Part model, mm, in its own coordinate system. Face numbers are marked on the shaded views. A direction names the side the tool comes from. Give positions to 0.01 mm unless a question says otherwise; leave off trailing zeros. Write each loop counter-clockwise with the first axis right and the second up, starting at its lowest first coordinate (ties: lowest second). Pieces come first, ordered by that corner, then holes. Notation, with made-up numbers: M 70,2 L 89,2 A14 ccw 89,26 Z; hole C -15.75,42 d5. An arc over 180 degrees is marked long. Answer as CSV lines item,"result". Start each with the question number.
Item 1: Band-saw the part on B-B, the plane z = 23. List the corners of the cut face in (x, y), then the cut area to 3 significant figures.
Item 2: Band-saw the part on D-D, the plane z = 9. List the corners of the cut face in (x, y), then the cut area to 3 significant figures.
Item 3: Band-saw the part on C-C, the plane x = 22.5. List the corners of the cut face in (y, z).
Item 4: Wall check: L1, parallel to Y at x = 39, z = 1; L2, parallel to Y at x = 28, z = 8; L3, parallel to Y at x = 44.5, z = 46.5. Give the ranges that are in metal, low to high. Write a range as from..to.
Item 5: Two-plate mould, pull along Y, no slides. Class the marked faces 5, 6 and 7: +Y half, -Y half, draft (parallel to the pull), parting line (faces both ways), or undercut.
Item 6: Pin check, flat tips, straight feed: pin 1 (16 mm diameter, centred on x = 12, z = 23, fed in from -Y); pin 2 (4.5 mm diameter, centred on x = 19.5, y = 24.5, fed in from +Z); pin 3 (1 mm diameter, centred on x = 43.5, y = 31, fed in from +Z). Stop position of each tip, or through.
Item 7: 3-axis set-ups, long thin cutter, end or side, ignore diameter. For the marked faces 1, 2, 3 and 4: which of +Z, -Z, +X, -X, +Y, -Y reach the whole face in a straight line?
Item 8: Band-saw the part on A-A, the plane y = 58. List the corners of the cut face in (x, z).
from build123d import *

# Parameters (mm, degrees)
F0_W           = 56
F0_H           = 66
F1_DEPTH       = 4
F3_D           = 7
F4_SIZE2       = 10
F4_SIZE        = 10
F5_SIZE2       = 16
F5_SIZE        = 16
F8_DEPTH       = 10
F8_DEPTH_BACK  = 10
F9_R           = 2
F11_R          = 5
F11_R_2        = 4
F12_DEPTH      = 20
F11_R_3        = 9.5
F13_DEPTH      = 1
F13_DEPTH_BACK = 21
F15_DEPTH      = 8
F15_DEPTH_BACK = 28
F10_W          = 12
F10_H          = 50
F16_DEPTH      = 61.001
F18_T4_DEPTH   = 56
F18_T9_DEPTH   = 61
F18_T15_DEPTH  = 56
F18_T20_DEPTH  = 61
F18_T26_DEPTH  = 56
F18_T31_DEPTH  = 61
F18_T37_DEPTH  = 56
F18_T42_DEPTH  = 61
F19_R          = 2


# Not quite as in the source:
# - a fillet or chamfer that OpenCascade refuses, or shapes differently, is made with other operations: its cross-section is extruded or revolved along the edge and cut away or added


with BuildPart() as f1:
    # F0 (on Top) → F1 (new body)
    with BuildSketch(Plane.XY):
        with Locations((28, 33)):
            Rectangle(F0_W, F0_H)
    extrude(amount=F1_DEPTH)

    # F3 (through all)
    with Locations(Plane.XY.offset(4)):
        with Locations((12, 58), (39, 58), (39, 8), (12, 8)):
            Hole(F3_D / 2)

    # F4
    f4_edges = [f1.edges().sort_by_distance(p)[0] for p in [
        (0, 66, 2),
        (0, 0, 2),
    ]]
    chamfer(f4_edges, length=F4_SIZE, length2=F4_SIZE2)

    # F5
    f5_edges = [f1.edges().sort_by_distance(p)[0] for p in [
        (56, 66, 2),
        (56, 0, 2),
    ]]
    chamfer(f5_edges, length=F5_SIZE, length2=F5_SIZE2)


with BuildPart() as f8:
    # F7 (on mid) → F8 (new body, two sides)
    with BuildSketch(Plane.XZ.offset(-33)) as f8_sk:
        with BuildLine():
            Line((0, 36), (0, 4))
            Line((0, 4), (56, 4))
            Line((56, 4), (60.6153846154, 15.0769230769))
            ThreePointArc((60.6153846154, 15.0769230769), (60.1602514717, 19.7735009811), (56, 22))
            Line((56, 22), (49, 36))
            Line((49, 36), (49, 41.5))
            ThreePointArc((49, 41.5), (39.5, 51), (30, 41.5))
            Line((30, 41.5), (30, 36))
            Line((30, 36), (0, 36))
        make_face()
    extrude(amount=-F8_DEPTH)
    extrude(f8_sk.sketch, amount=F8_DEPTH_BACK)

    # F9
    f9_edges = [f8.edges().sort_by_distance(p)[0] for p in [
        (30, 33, 36),
        (49, 33, 36),
        (0, 33, 36),
    ]]
    fillet(f9_edges, radius=F9_R)

    # F11 (on face) → F12 (cut, through all)
    with BuildSketch(Plane.XZ.offset(-23)):
        with Locations((12, 23)):
            Circle(F11_R)
        with Locations((39.5, 41.5)):
            Circle(F11_R_2)
    extrude(amount=-F12_DEPTH, mode=Mode.SUBTRACT)

    # F11 (on face) → F13 (join, two sides)
    with BuildSketch(Plane.XZ.offset(-23)) as f13_sk:
        with Locations((12, 23)):
            Circle(F11_R_3)
        with Locations((12, 23)):
            Circle(F11_R, mode=Mode.SUBTRACT)
        with BuildLine():
            ThreePointArc((30, 41.5), (39.5, 32), (49, 41.5))
            ThreePointArc((49, 41.5), (39.5, 51), (30, 41.5))
        make_face()
        with Locations((39.5, 41.5)):
            Circle(F11_R_2, mode=Mode.SUBTRACT)
    extrude(amount=F13_DEPTH)
    extrude(f13_sk.sketch, amount=-F13_DEPTH_BACK)

    # F14 (on face) → F15 (join, two sides)
    with BuildSketch(Plane.XZ.offset(-23)) as f15_sk:
        with BuildLine():
            ThreePointArc((60.6153846154, 15.0769230769), (60.9029033785, 16.0194193243), (61, 17))
            ThreePointArc((61, 17), (59.5355339059, 20.5355339059), (56, 22))
            ThreePointArc((56, 22), (51.8397485283, 14.2264990189), (60.6153846154, 15.0769230769))
        make_face()
    extrude(amount=F15_DEPTH)
    extrude(f15_sk.sketch, amount=-F15_DEPTH_BACK)

    # F10 (on face) → F16 (cut, through all)
    with BuildSketch(Plane(origin=(0, 0, 0), x_dir=(0, -1, 0), z_dir=(-1, 0, 0))):
        with Locations((-33, 29)):
            Rectangle(F10_W, F10_H)
    extrude(amount=-F16_DEPTH, mode=Mode.SUBTRACT)


with BuildPart() as f1_1:
    add(f1.part)

    # F17: union F8
    add(f8.part)

    # F18: fillet of radius 2 on 4 edges, made by hand


with BuildPart() as f18_tool2:
    # F18_s3 → F18_t4 (new body)
    with BuildSketch(Plane.YZ):
        with BuildLine():
            ThreePointArc((21, 4), (22.4142135624, 4.5857864376), (23, 6))
            Line((23, 6), (23, 4))
            Line((23, 4), (21, 4))
        make_face()
    extrude(amount=F18_T4_DEPTH)

    split(bisect_by=Plane(origin=(46.2958579882, 0, -19.2899408284), x_dir=(0, 1, 0), z_dir=(-0.9230769231, 0, 0.3846153846)), keep=Keep.TOP)


with BuildPart() as f1_2:
    add(f1_1.part)

    # F18_t1: union F18_tool2
    add(f18_tool2.part)


with BuildPart() as f18_tool7:
    # F18_s8 → F18_t9 (new body)
    with BuildSketch(Plane.YZ):
        with BuildLine():
            ThreePointArc((21, 4), (22.4142135624, 4.5857864376), (23, 6))
            Line((23, 6), (23, 4))
            Line((23, 4), (21, 4))
        make_face()
    extrude(amount=F18_T9_DEPTH)

    split(bisect_by=Plane.YZ.offset(56), keep=Keep.TOP)

    split(bisect_by=Plane(origin=(46.2958579882, 0, -19.2899408284), x_dir=(0, 1, 0), z_dir=(-0.9230769231, 0, 0.3846153846)), keep=Keep.TOP)


with BuildPart() as f1_3:
    add(f1_2.part)

    # F18_t6: union F18_tool7
    add(f18_tool7.part)


with BuildPart() as f18_tool13:
    # F18_s14 → F18_t15 (new body)
    with BuildSketch(Plane.YZ):
        with BuildLine():
            ThreePointArc((37, 4), (38.4142135624, 4.5857864376), (39, 6))
            Line((39, 6), (39, 4))
            Line((39, 4), (37, 4))
        make_face()
    extrude(amount=F18_T15_DEPTH)

    split(bisect_by=Plane(origin=(46.2958579882, 0, -19.2899408284), x_dir=(0, 1, 0), z_dir=(-0.9230769231, 0, 0.3846153846)), keep=Keep.TOP)


with BuildPart() as f1_4:
    add(f1_3.part)

    # F18_t12: union F18_tool13
    add(f18_tool13.part)


with BuildPart() as f18_tool18:
    # F18_s19 → F18_t20 (new body)
    with BuildSketch(Plane.YZ):
        with BuildLine():
            ThreePointArc((37, 4), (38.4142135624, 4.5857864376), (39, 6))
            Line((39, 6), (39, 4))
            Line((39, 4), (37, 4))
        make_face()
    extrude(amount=F18_T20_DEPTH)

    split(bisect_by=Plane.YZ.offset(56), keep=Keep.TOP)

    split(bisect_by=Plane(origin=(46.2958579882, 0, -19.2899408284), x_dir=(0, 1, 0), z_dir=(-0.9230769231, 0, 0.3846153846)), keep=Keep.TOP)


with BuildPart() as f1_5:
    add(f1_4.part)

    # F18_t17: union F18_tool18
    add(f18_tool18.part)


with BuildPart() as f18_tool24:
    # F18_s25 → F18_t26 (new body)
    with BuildSketch(Plane.YZ):
        with BuildLine():
            ThreePointArc((45, 4), (43.5857864376, 4.5857864376), (43, 6))
            Line((43, 6), (43, 4))
            Line((43, 4), (45, 4))
        make_face()
    extrude(amount=F18_T26_DEPTH)

    split(bisect_by=Plane(origin=(46.2958579882, 0, -19.2899408284), x_dir=(0, 1, 0), z_dir=(-0.9230769231, 0, 0.3846153846)), keep=Keep.TOP)


with BuildPart() as f1_6:
    add(f1_5.part)

    # F18_t23: union F18_tool24
    add(f18_tool24.part)


with BuildPart() as f18_tool29:
    # F18_s30 → F18_t31 (new body)
    with BuildSketch(Plane.YZ):
        with BuildLine():
            ThreePointArc((45, 4), (43.5857864376, 4.5857864376), (43, 6))
            Line((43, 6), (43, 4))
            Line((43, 4), (45, 4))
        make_face()
    extrude(amount=F18_T31_DEPTH)

    split(bisect_by=Plane.YZ.offset(56), keep=Keep.TOP)

    split(bisect_by=Plane(origin=(46.2958579882, 0, -19.2899408284), x_dir=(0, 1, 0), z_dir=(-0.9230769231, 0, 0.3846153846)), keep=Keep.TOP)


with BuildPart() as f1_7:
    add(f1_6.part)

    # F18_t28: union F18_tool29
    add(f18_tool29.part)


with BuildPart() as f18_tool35:
    # F18_s36 → F18_t37 (new body)
    with BuildSketch(Plane.YZ):
        with BuildLine():
            ThreePointArc((29, 4), (27.5857864376, 4.5857864376), (27, 6))
            Line((27, 6), (27, 4))
            Line((27, 4), (29, 4))
        make_face()
    extrude(amount=F18_T37_DEPTH)

    split(bisect_by=Plane(origin=(46.2958579882, 0, -19.2899408284), x_dir=(0, 1, 0), z_dir=(-0.9230769231, 0, 0.3846153846)), keep=Keep.TOP)


with BuildPart() as f1_8:
    add(f1_7.part)

    # F18_t34: union F18_tool35
    add(f18_tool35.part)


with BuildPart() as f18_tool40:
    # F18_s41 → F18_t42 (new body)
    with BuildSketch(Plane.YZ):
        with BuildLine():
            ThreePointArc((29, 4), (27.5857864376, 4.5857864376), (27, 6))
            Line((27, 6), (27, 4))
            Line((27, 4), (29, 4))
        make_face()
    extrude(amount=F18_T42_DEPTH)

    split(bisect_by=Plane.YZ.offset(56), keep=Keep.TOP)

    split(bisect_by=Plane(origin=(46.2958579882, 0, -19.2899408284), x_dir=(0, 1, 0), z_dir=(-0.9230769231, 0, 0.3846153846)), keep=Keep.TOP)


with BuildPart() as f1_9:
    add(f1_8.part)

    # F18_t39: union F18_tool40
    add(f18_tool40.part)

    # F19
    f19_edges = [f1_9.edges().sort_by_distance(p)[0] for p in [
        (40, 0, 2),
        (56, 16, 2),
        (10, 0, 2),
        (56, 50, 2),
        (40, 66, 2),
        (10, 66, 2),
        (0, 56, 2),
        (0, 10, 2),
    ]]
    fillet(f19_edges, radius=F19_R)


solid = f1_9.part
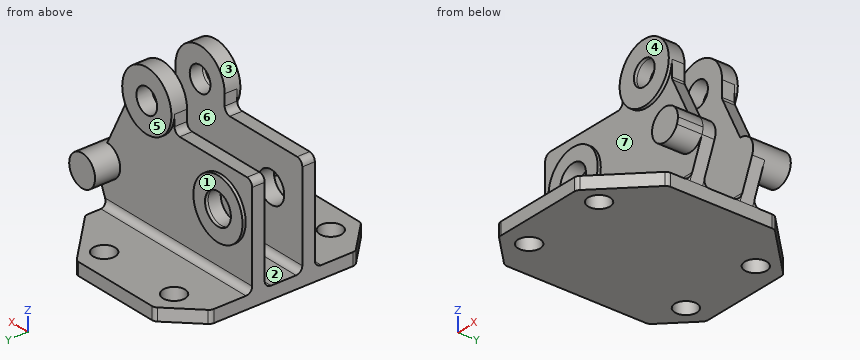
Output:
1,outline,"M 0,23 L 2.5,23 L 2.5,22 L 7,22 L 7,27 L 0,27 Z; M 0,39 L 7,39 L 7,44 L 2.5,44 L 2.5,43 L 0,43 Z; M 17,22 L 21.5,22 L 21.5,23 L 55.5,23 L 55.5,27 L 17,27 Z; M 17,39 L 55.5,39 L 55.5,43 L 21.5,43 L 21.5,44 L 17,44 Z"
1,area,"382 mm²"
2,outline,"M 0,23 L 58.08,23 L 58.08,27 L 0,27 Z; M 0,39 L 58.08,39 L 58.08,43 L 0,43 Z"
2,area,"465 mm²"
3,outline,"M 0,0 L 66,0 L 66,4 L 45,4 A2 cw 43,6 L 43,36 L 39,36 L 39,6 A2 cw 37,4 L 29,4 A2 cw 27,6 L 27,36 L 23,36 L 23,6 A2 cw 21,4 L 0,4 Z"
4,L1,"0..4.5, 11.5..54.5, 61.5..66"
4,L2,"23..27, 39..43"
4,L3,"22..27, 39..44"
5,face 5,"+Y half"
5,face 6,"undercut"
5,face 7,"-Y half"
6,pin 1,"y = 22"
6,pin 2,"z = 36"
6,pin 3,"z = 4"
7,face 1,"+Z, -X, +Y"
7,face 2,"+Z, +X, -X"
7,face 3,"-Y"
7,face 4,"+Z, +X, -X, -Y"
8,outline,"M 2,0 L 8.5,0 L 8.5,4 L 2,4 Z; M 15.5,0 L 35.5,0 L 35.5,4 L 15.5,4 Z; M 42.5,0 L 48,0 L 48,4 L 42.5,4 Z"
